```python
from build123d import *

# Parameters (mm, degrees)
SKETCH1_R           = 85
SKETCH1_R_2         = 70
BOSS_EXTRUDE1_DEPTH = 10
SKETCH2_R           = 75
CUT_EXTRUDE2_DEPTH  = 5
SKETCH3_R           = 1.5
CUT_EXTRUDE3_DEPTH  = 10
CIRPATTERN1_COUNT   = 6
FILLET1_R           = 1


with BuildPart() as part:
    # Sketch1 → Boss-Extrude1 (new body)
    with BuildSketch(Plane.XY):
        Circle(SKETCH1_R)
        Circle(SKETCH1_R_2, mode=Mode.SUBTRACT)
    extrude(amount=BOSS_EXTRUDE1_DEPTH)

    # Sketch2 → Cut-Extrude2 (cut)
    with BuildSketch(Plane.XY):
        Circle(SKETCH2_R)
    extrude(amount=CUT_EXTRUDE2_DEPTH, mode=Mode.SUBTRACT)

    # Sketch3 → Cut-Extrude3 (cut)
    with BuildSketch(Plane(origin=(0, 0, 0), x_dir=(-1, 0, 0), z_dir=(0, 0, -1))):
        with Locations((0, 80)):
            Circle(SKETCH3_R)
    cut_extrude3 = extrude(amount=-CUT_EXTRUDE3_DEPTH, mode=Mode.SUBTRACT)

    # CirPattern1: Cut-Extrude3 ×6 about axis
    cirpattern1_axis = Axis((0, 0, 0), (0, 0, 1))
    for i in range(1, CIRPATTERN1_COUNT):
        add(cut_extrude3.rotate(cirpattern1_axis, i * 360 / CIRPATTERN1_COUNT), mode=Mode.SUBTRACT)

    # Fillet1
    fillet1_edges = [part.edges().sort_by_distance(p)[0] for p in [
        (-75, 0, 0),
        (-85, 0, 10),
    ]]
    fillet(fillet1_edges, radius=FILLET1_R)


solid = part.part
```
Here's how the part is built. I have some questions about the finished solid (model axes, mm). A direction names the side the tool comes from. Coordinates: 2 decimals unless noted, no trailing zeros. Order: outer loops, then holes, each group sorted by start corner. A loop starts at its lowest first (then second) coordinate and runs counter-clockwise, first axis right, second up. Notation, with made-up numbers: M 60,-11.5 L 79,-11.5 A22 ccw 79,8.5 Z; hole C -18,8.5 d7. An arc over 180 degrees is marked long. Answer as a JSON object with one key per item and string values. Group by question number.
(1) For pin 1 (2 mm diameter, centred on x = 47, z = 3, fed in from +Y); pin 2 (6 mm diameter, centred on x = 64, z = 7, fed in from -Y); pin 3 (4 mm diameter, centred on x = -69.28, y = -40, fed in from +Z); pin 4 (1 mm diameter, centred on x = 26.5, z = 3, fed in from +Y), each with a flat end and sliding along its axis, tell me the tip position at first contact or that it passes through.
(2) Suppose I cut it at A-A, the plane y = 0. Please give me the cut outline in (x, z), then the cut area to 3 significant figures.
(3) I need wall thicknesses on probe 1 along Y at (x, z) = (0, 7.9); probe 2 along Y at (x, z) = (0, 2); probe 3 along Z at (x, y) = (36.5, -62). Which ranges of each line are inside material? Lowest first, please.
(4) If we mould it in two halves opening along Y, with no side actions, what happens to faces 1 (the face through (-19, -68, 10)), 2 (the face through (-9.764, 74.362, 2.972)), 3 (the face through (-67.453, -51.721, 4.437))? For each: released by +Y, released by -Y, zero draft, split by the parting line, or undercut.
(5) Which directions (+Z, -Z, +X, -X, +Y, -Y) give clear straight access to the entire face, cutting with the end or side of a thin tool? Please do faces 4 (the face through (50, -50, 5)), 5 (the face through (-63, -44, 0)).
(6) Suppose I cut it at B-B, the plane z = 3.5. Please give me the cut outline in (x, y).
Values found:
{
 "1": {"pin 1": "stops at y = 71.48", "pin 2": "stops at y = -59.19", "pin 3": "stops at z = 10", "pin 4": "stops at y = 80.93"},
 "2": {"outline": "M -85,0 L -76,0 A1 ccw -75,1 L -75,5 L -70,5 L -70,10 L -84,10 A1 ccw -85,9 Z; M 70,5 L 75,5 L 75,1 A1 ccw 76,0 L 85,0 L 85,9 A1 ccw 84,10 L 70,10 Z", "area": "249 mm^2"},
 "3": {"probe 1": "y = -85 to -81.5, -78.5 to -70, 70 to 78.5, 81.5 to 85", "probe 2": "y = -85 to -81.5, -78.5 to -75, 75 to 78.5, 81.5 to 85", "probe 3": "z = 5 to 10"},
 "4": {"face 1": "zero draft", "face 2": "undercut", "face 3": "split by the parting line"},
 "5": {"face 4": "-Z", "face 5": "-Z, +X, -X, +Y, -Y"},
 "6": {"outline": "C 0,0 d170; hole C 0,0 d150; hole C -69.28,-40 d3; hole C -69.28,40 d3; hole C 0,-80 d3; hole C 0,80 d3; hole C 69.28,-40 d3; hole C 69.28,40 d3"}
}
